```python
from build123d import *

# Parameters (mm, degrees)
BLANKSKE_W               = 877.6
BLANKSKE_H               = 168.84
BLANK_DEPTH              = 120
TOOTHCUTSIM_DEPTH        = 902.714314847
TEETHCUTS_COUNT          = 21
TEETHCUTS_PITCH          = 43.9822971
SKETCH_1_R               = 29
SKETCH_1_R_2             = 20
CUT_EXTRUDE_2_DEPTH      = 60
SKETCH_2_R               = 21
CUT_EXTRUDE_3_DEPTH      = 60
HOLE_WIZARD_1_AT_2_COUNT = 2
HOLE_WIZARD_1_AT_2_PITCH = 584


with BuildPart() as part:
    # BlankSke → Blank (new body)
    with BuildSketch(Plane.XY):
        with Locations((438.8, 84.42)):
            Rectangle(BLANKSKE_W, BLANKSKE_H)
    extrude(amount=-BLANK_DEPTH)

    # TooCutSkeSim → ToothCutSim (cut, through all)
    with BuildSketch(Plane.XY):
        Polygon((5.946095175, 137.34), (-5.946095175, 137.34), (-17.420402399, 168.8654), (17.420402399, 168.8654), align=None)
    toothcutsim = extrude(amount=-TOOTHCUTSIM_DEPTH, mode=Mode.SUBTRACT)

    # TeethCuts: ToothCutSim ×21
    with Locations(*[(i * TEETHCUTS_PITCH, 0, 0) for i in range(1, TEETHCUTS_COUNT)]):
        add(toothcutsim, mode=Mode.SUBTRACT)

    # 草图1 → 切除-拉伸2 (cut)
    with BuildSketch(Plane.XY):
        with Locations((48, 58)):
            Circle(SKETCH_1_R)
        with Locations((146, 58)):
            Circle(SKETCH_1_R_2)
        with Locations((243, 58)):
            Circle(SKETCH_1_R)
        with Locations((438, 58)):
            Circle(SKETCH_1_R)
        with Locations((633, 58)):
            Circle(SKETCH_1_R)
        with Locations((730, 58)):
            Circle(SKETCH_1_R_2)
        with Locations((828, 58)):
            Circle(SKETCH_1_R)
    extrude(amount=-CUT_EXTRUDE_2_DEPTH, mode=Mode.SUBTRACT)

    # 草图2 → 切除-拉伸3 (cut)
    with BuildSketch(Plane.XY.offset(-60)):
        with Locations((48, 58)):
            Circle(SKETCH_2_R)
        with Locations((243, 58)):
            Circle(SKETCH_2_R)
        with Locations((438, 58)):
            Circle(SKETCH_2_R)
        with Locations((633, 58)):
            Circle(SKETCH_2_R)
        with Locations((828, 58)):
            Circle(SKETCH_2_R)
    extrude(amount=-CUT_EXTRUDE_3_DEPTH, mode=Mode.SUBTRACT)

    # 草图6 → 孔1 (revolve, cut)
    with BuildSketch(Plane(origin=(146, 58, -60), x_dir=(0, -1, 0), z_dir=(1, 0, 0))):
        Polygon((0, 0), (0, 60), (10, 60), (15, 0), align=None)
    hole_wizard_1 = revolve(axis=Axis((146, 58, -170), (0, 0, 1)), mode=Mode.SUBTRACT)

    # 孔1 at 2: 孔1 ×2
    with Locations(*[(i * HOLE_WIZARD_1_AT_2_PITCH, 0, 0) for i in range(1, HOLE_WIZARD_1_AT_2_COUNT)]):
        add(hole_wizard_1, mode=Mode.SUBTRACT)


solid = part.part
```
For this review, take the finished solid that the model builds, in its own axes (mm). A direction names the side the tool comes from. Coordinates: 2 decimals unless noted, no trailing zeros. Answer as a JSON object with one key per item and string values. Group by question number.
1. For probe 1 along Y at (x, z) = (243, -96.5); probe 2 along Y at (x, z) = (438, -99); probe 3 along X at (y, z) = (44, -84), list the stretches that pass through material, from the lowest coordinate up.
2. For faces 1 (the flat face through (187.69, 153.31, -59.16)), 2 (the cylindrical face through (227.52, 72.19, -89.58)), 3 (the cylindrical face through (660.66, 66.71, -29.58)), list the 3-axis set-ups (+Z, -Z, +X, -X, +Y, -Y) from which the entire face can be reached by the end or side of a thin tool; tool diameter is ignored.
3. The part is to be moulded in two halves that separate along Y. For faces 4 (the cylindrical face through (126.02, 58.88, -29.58)), 5 (the flat face through (451.58, 153.31, -59.16)), say which applies: pulls with the +Y half, pulls with the -Y half, needs draft (parallel to the pull), parting line crosses it, or undercut.
4. We need section A-A on y = 58. Give the number of separate pieces and of enclosed holes in the cut face, then the cut area to 3 significant figures.
5. Clearance check with flat-ended pins moving along their axes: P1, Ø6, axis at x = 42, z = -74, coming from the +Y side; P2, Ø1, axis at x = 94.5, z = -21.5, coming from the -Y side. State where each tip first meets the part, or that it passes through.
Final values:
{
 "1": {"probe 1": "0 to 37, 79 to 168.84", "probe 2": "0 to 37, 79 to 137.34", "probe 3": "0 to 32.35, 63.65 to 227.35, 258.65 to 422.35, 453.65 to 617.35, 648.65 to 812.35, 843.65 to 877.6"},
 "2": {"face 1": "+Z, -Z, +Y", "face 2": "+Z, -Z", "face 3": "+Z"},
 "3": {"face 4": "undercut", "face 5": "pulls with the +Y half"},
 "4": {"separate pieces": "8", "enclosed holes": "0", "area": "67,500 mm²"},
 "5": {"P1": "y = 137.34", "P2": "y = 0"}
}
